Design review of the part built by this model. Coordinates are the model's own, in mm. Face numbers are marked on the shaded views. Give positions to 0.01 mm unless a question says otherwise; leave off trailing zeros. Write each loop counter-clockwise with the first axis right and the second up, starting at its lowest first coordinate (ties: lowest second). Pieces come first, ordered by that corner, then holes. Notation, with made-up numbers: M -20.5,-3 L 28.5,-3 A29 ccw 28.5,32 Z; hole C -39,64.25 d2. An arc over 180 degrees is marked long. Answer in a Markdown table with one row per item.
```python
from build123d import *

# Parameters (mm, degrees)
SCALE1_SCALE       = 649.76746201
SHELL2_T           = 5.588
SKETCH3_R          = 101.6
SKETCH3_R_2        = 66.04
CUT_EXTRUDE2_DEPTH = 535.742534837
CUT_EXTRUDE3_START = -41.91
SKETCH4_R          = 92.04718224
CUT_EXTRUDE3_DEPTH = 41.91
CUT_EXTRUDE4_START = -12.7
SKETCH5_R          = 73.005644817
CUT_EXTRUDE4_DEPTH = 50.8
SKETCH6_W          = 424.059423161
SKETCH6_H          = 690.342462677
CUT_EXTRUDE5_DEPTH = 250.634607617


with BuildPart() as part:
    # Sketch1 → Revolve2 (revolve)
    with BuildSketch(Plane.XY, mode=Mode.PRIVATE) as revolve2_sk:
        with BuildLine():
            Line((0.30325, 0.129), (-0.275595218, 0.129))
            ThreePointArc((-0.275595218, 0.129), (-0.3184401, 0.116916493), (-0.348657753, 0.084227221))
            Line((-0.348657753, 0.084227221), (-0.372858421, 0.036730735))
            ThreePointArc((-0.372858421, 0.036730735), (-0.374701425, 0.034736985), (-0.377314576, 0.034))
            Line((-0.377314576, 0.034), (-0.40125, 0.034))
            Line((-0.40125, 0.034), (-0.40125, 0))
            Line((-0.40125, 0), (0.40125, 0))
            Line((0.40125, 0), (0.40125, 0.000587576))
            ThreePointArc((0.40125, 0.000587576), (0.399958659, 0.015347671), (0.396123873, 0.029659288))
            Line((0.396123873, 0.029659288), (0.379365102, 0.075703632))
            ThreePointArc((0.379365102, 0.075703632), (0.349709691, 0.114351316), (0.30325, 0.129))
        make_face()
    revolve(revolve2_sk.sketch.rotate(Axis((-0.40125, 0, 0), (1, 0, 0)), 90), axis=Axis((-0.40125, 0, 0), (1, 0, 0)))


with BuildPart() as part_1:
    # Scale1: scaled about (0, 0, 0)
    add(part.part.scale(SCALE1_SCALE))

    # Shell2 (no face opened: a closed hollow body)
    add(offset(amount=-SHELL2_T, mode=Mode.PRIVATE), mode=Mode.SUBTRACT)

    # Sketch3 → Cut-Extrude2 (cut, through all)
    with BuildSketch(Plane.ZY.offset(260.719194132)):
        Circle(SKETCH3_R)
        with Locations(Location((0, 0, 0), (0, 0, 180))):
            Circle(SKETCH3_R_2, mode=Mode.SUBTRACT)
    extrude(amount=-CUT_EXTRUDE2_DEPTH, mode=Mode.SUBTRACT)


with BuildPart() as body_2:
    # of the pieces the cut leaves, the one that is kept (cut_extrude2_keep)
    add(part_1.part.solids().sort_by_distance((-218.803671245, 0, 66.04))[0])

    # Sketch4 → Cut-Extrude3 (cut)
    with BuildSketch(Plane.ZY.offset(260.719194132).offset(CUT_EXTRUDE3_START)):
        Circle(SKETCH4_R)
    extrude(amount=-CUT_EXTRUDE3_DEPTH, mode=Mode.SUBTRACT)

    # Sketch5 → Cut-Extrude4 (cut)
    with BuildSketch(Plane(origin=(-218.809194132, 0, 0), x_dir=(0, 0, -1), z_dir=(1, 0, 0)).offset(CUT_EXTRUDE4_START)):
        Circle(SKETCH5_R)
    extrude(amount=-CUT_EXTRUDE4_DEPTH, mode=Mode.SUBTRACT)

    # Sketch6 → Cut-Extrude5 (cut, through all)
    with BuildSketch(Plane.XY):
        with Locations((-333.697276698, 135.370996171)):
            Rectangle(SKETCH6_W, SKETCH6_H)
    extrude(amount=-CUT_EXTRUDE5_DEPTH, mode=Mode.SUBTRACT)


solid = body_2.part
```
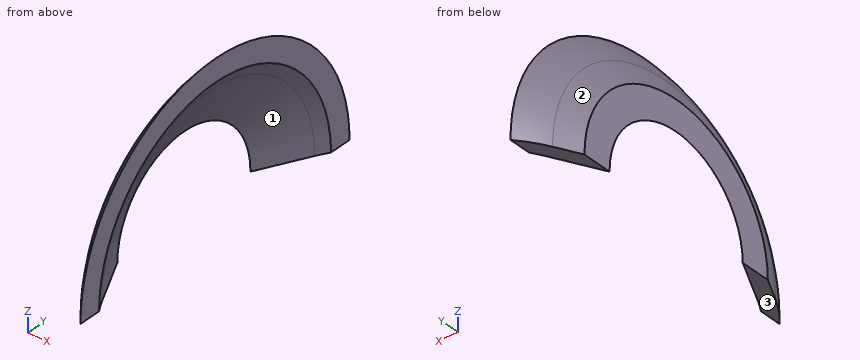
1) To check wall thickness, follow probe 1 along Y at (x, z) = (-230, 13); probe 2 along Y at (x, z) = (-226, 11.5); probe 3 along Z at (x, y) = (-229.25, 10). State the ranges of each line that lie inside material, in increasing order. Write a range as [from, to].
Geometry says:
| item | result |
|---|---|
| probe 1 | [-46.15, -33.19], [33.19, 46.15] |
| probe 2 | [-54.57, -41.94], [41.94, 54.57] |
| probe 3 | [35.74, 48.4] |
2) Add section A-A (x = -230). Write out the cut boundary in (y, z).
Geometry says:
| item | result |
|---|---|
| outline | M -47.95,0 L -35.64,0 A35.64 cw 35.64,0 L 47.95,0 A47.95 ccw Z |
3) Insertion check: P1, Ø1, axis at x = -224.5, y = -7, coming from the -Z side; P2, Ø2, axis at y = -45, z = 12, coming from the +X side; P3, Ø8, axis at y = 49.5, z = 17, coming from the -X side. Each pin has a flat end and moves straight along its axis. Give the tip position at first contact, or say it passes through.
Geometry says:
| item | result |
|---|---|
| P1 | z = 44.91 |
| P2 | x = -223.92 |
| P3 | x = -229.8 |
4) The part is to be moulded in two halves that separate along Y. For the marked faces 1, 2 and 3, say which applies: released by +Y, released by -Y, zero draft, split by the parting line, or undercut.
Geometry says:
| item | result |
|---|---|
| face 1 | undercut |
| face 2 | split by the parting line |
| face 3 | zero draft |
